```python
from build123d import *

# Parameters (mm, degrees)
EXTRUDE004_DEPTH  = 10
CYLINDER024_R     = 2
CYLINDER024_DEPTH = 20
EXTRUDE003_DEPTH  = 20


with BuildPart() as extrude004:
    # Sketch006 → Extrude004 (new body)
    with BuildSketch(Plane(origin=(0, 20, 0), x_dir=(-1, 0, 0), z_dir=(0, 1, 0))):
        Polygon((24, -38), (32, -30), (33, -30), (33, -39), (11, -39), (11, -30), (12, -30), (20, -38), align=None)
    extrude(amount=-EXTRUDE004_DEPTH)


with BuildPart() as extrude004_1:
    # Extrude004 placement: moved
    add(extrude004.part.moved(Location((0, -23, 0))))


with BuildPart() as fusion005:
    # Cylinder024 → Cylinder024 (new body)
    with BuildSketch(Plane(origin=(-22, 0, -32.5), x_dir=(1, 0, 0), z_dir=(0, -1, 0))):
        Circle(CYLINDER024_R)
    extrude(amount=CYLINDER024_DEPTH)

    # Fusion005: union Extrude004
    add(extrude004_1.part)


with BuildPart() as body001:
    # Sketch005 → Extrude003 (new body)
    with BuildSketch(Plane(origin=(-80, 0, 0), x_dir=(0, -1, 0), z_dir=(-1, 0, 0))):
        with BuildLine():
            Line((9.222057, -26.966565), (9.222057, -37.966565))
            Line((9.222057, -37.966565), (6.222057, -37.966565))
            Line((6.222057, -37.966565), (6.222057, -27.540914))
            ThreePointArc((2.629328, -21.56221), (3.857128, -24.893224), (6.222057, -27.540914))
            Line((1.5, -11.75), (2.629328, -21.56221))
            Line((1.5, -6.75), (1.5, -11.75))
            Line((12, -6.75), (1.5, -6.75))
            Line((12, -8.75), (12, -6.75))
            Line((12, -8.75), (3.5, -8.75))
            Line((3.5, -8.75), (3.5, -11.75))
            Line((3.5, -11.75), (4.602099, -21.233313))
            ThreePointArc((4.602099, -21.233313), (6.160095, -24.705901), (9.222057, -26.966565))
        make_face()
    extrude(amount=-EXTRUDE003_DEPTH)


with BuildPart() as body001_1:
    # Extrude003 placement: moved
    add(body001.part.moved(Location((48, 0, 0))))

    # Cut004: cut Fusion005
    add(fusion005.part, mode=Mode.SUBTRACT)


with BuildPart() as part_mirroring001:
    # Part__Mirroring001: instance of Body001
    add(body001_1.part.mirror(Plane(origin=(0, -12, 0), x_dir=(1, 0, 0), z_dir=(0, 1, 0))))


solid = part_mirroring001.part
```
Read the model definition and answer for the solid it produces. Units are mm, in the model's axes. A direction names the side the tool comes from. Give positions to 0.01 mm unless a question says otherwise; leave off trailing zeros. Order: outer loops, then holes, each group sorted by start corner. A loop starts at its lowest first (then second) coordinate and runs counter-clockwise, first axis right, second up.
(1) Find section C-C (y = -16.75). Give the vertices of the cut face in (x, z).
(2) Given pin 1 (3 mm diameter, centred on x = -21.5, z = -35, fed in from -Y); pin 2 (5 mm diameter, centred on x = -27, z = -23, fed in from -Y); pin 3 (3 mm diameter, centred on x = -22.5, z = -18, fed in from +Y), each flat-ended and moving along its own axis, determine where each tip first touches the part or whether it passes through.
(3) Find section A-A (x = -22). Give the vertices of the cut face in (y, z).
(4) For faces 4 (the flat face through (-22, -14.778, -30)), 5 (the flat face through (-22, -20.5, -10)), 6 (the flat face through (-24.4, -17.778, -31.7)), determine the directions among +Z, -Z, +X, -X, +Y, -Y from which every point of the face is accessible in a straight line to the end or side of a thin tool.
(5) Find section D-D (y = -13.5). Give the vertices of the cut face in (x, z), plus the area to 3 significant figures.
(6) Straight lines are drawn through the part: L1, parallel to Z at x = -22, y = -16.2; L2, parallel to Z at x = -22, y = -16.5; L3, parallel to Z at x = -20.25, y = -13.75. For each, find the intervals that lie inside material, in ascending order.
(7) Find section B-B (z = -32.5). Give the vertices of the cut face in (x, y), plus the area to 3 significant figures.
(8) For a pull along X with two mould halves and no side action, classify faces 1 (the cylindrical face through (-22.434, -16.299, -34.452)), 2 (the flat face through (-22, -17, -6.75)), 3 (the flat face through (-32, -20.3, -16.6)) as released by +X, released by -X, zero draft, split by the parting line, or undercut.
Result sheet:
1. outline: (-32, -30) - (-24.03, -37.97) - (-19.97, -37.97) - (-12, -30) - (-12, -25.8) - (-32, -25.8) - close; (-32, -8.75) - (-12, -8.75) - (-12, -6.75) - (-32, -6.75) - close; hole circle Ø4 at (-22, -32.5)
2. pin 1: stops at y = -17.78
2. pin 2: stops at y = -21.49
2. pin 3: stops at y = -19.6
3. outline: (-22.5, -11.75) - (-21.37, -21.56) arc R9.5 ccw to (-17.78, -27.54) - (-17.78, -30.5) - (-14.78, -30.5) - (-14.78, -26.97) arc R7.5 cw to (-19.4, -21.23) - (-20.5, -11.75) - (-20.5, -8.75) - (-12, -8.75) - (-12, -6.75) - (-22.5, -6.75) - close; (-17.78, -37.97) - (-14.78, -37.97) - (-14.78, -34.5) - (-17.78, -34.5) - close
4. face 4: -Z, +X, -X, +Y
4. face 5: +X, -X, +Y
4. face 6: -Z, +X, -X, -Y
5. outline: (-32, -8.75) - (-12, -8.75) - (-12, -6.75) - (-32, -6.75) - close
5. area: 40.0 mm2
6. L1: z = -37.97 to -34.5, -30.5 to -26.21, -8.75 to -6.75
6. L2: z = -37.97 to -34.5, -30.5 to -26, -8.75 to -6.75
6. L3: z = -8.75 to -6.75
7. outline: (-29.5, -17.78) - (-24, -17.78) - (-24, -14.78) - (-29.5, -14.78) - close; (-20, -17.78) - (-14.5, -17.78) - (-14.5, -14.78) - (-20, -14.78) - close
7. area: 33.0 mm2
8. face 1: undercut
8. face 2: zero draft
8. face 3: released by -X
